from build123d import *

# Parameters (mm, degrees)
SKETCH1_R               = 18
BOSS_EXTRUDE1_DEPTH     = 7.5
CUT_EXTRUDE1_DEPTH      = 8.5
SKETCH3_R               = 6
BOSS_EXTRUDE2_DEPTH     = 2
SKETCH3_3_W             = 2.25
SKETCH3_3_H             = 1.5
CUT_EXTRUDE2_DEPTH      = 3
CUT_EXTRUDE2_DEPTH_BACK = 16
CIRPATTERN1_COUNT       = 16


with BuildPart() as part:
    # Sketch1 → Boss-Extrude1 (new body, symmetric)
    with BuildSketch(Plane.XY):
        Circle(SKETCH1_R)
    extrude(amount=BOSS_EXTRUDE1_DEPTH, both=True)

    # Sketch2 → Cut-Extrude1 (cut, symmetric)
    with BuildSketch(Plane.XY):
        with BuildLine():
            ThreePointArc((-2.51847991, 17.822941927), (-1.502149502, 15.735029188), (-1.035799814, 13.460205004))
            ThreePointArc((-1.035799814, 13.460205004), (0, 13.5), (1.035799814, 13.460205004))
            ThreePointArc((1.035799814, 13.460205004), (1.502149502, 15.735029188), (2.51847991, 17.822941927))
            ThreePointArc((2.51847991, 17.822941927), (0, 18), (-2.51847991, 17.822941927))
        make_face()
    cut_extrude1 = extrude(amount=CUT_EXTRUDE1_DEPTH, both=True, mode=Mode.SUBTRACT)

    # Sketch3 → Boss-Extrude2 (add)
    with BuildSketch(Plane.XY.offset(7.5)):
        Circle(SKETCH3_R)
        with BuildLine():
            ThreePointArc((1.125, 4.357106264), (0, -4.5), (-1.125, 4.357106264))
            Line((-1.125, 4.357106264), (-1.125, 5.107106264))
            Line((-1.125, 5.107106264), (1.125, 5.107106264))
            Line((1.125, 5.107106264), (1.125, 4.357106264))
        make_face(mode=Mode.SUBTRACT)
    extrude(amount=BOSS_EXTRUDE2_DEPTH)

    # Sketch3<3> → Cut-Extrude2 (cut, two sides)
    with BuildSketch(Plane.XY.offset(7.5)) as cut_extrude2_sk:
        with BuildLine():
            Line((1.125, 3.607106264), (-1.125, 3.607106264))
            Line((-1.125, 3.607106264), (-1.125, 4.357106264))
            ThreePointArc((-1.125, 4.357106264), (0, -4.5), (1.125, 4.357106264))
            Line((1.125, 4.357106264), (1.125, 3.607106264))
        make_face()
        with Locations((0, 4.357106264)):
            Rectangle(SKETCH3_3_W, SKETCH3_3_H)
    extrude(amount=CUT_EXTRUDE2_DEPTH, mode=Mode.SUBTRACT)
    extrude(cut_extrude2_sk.sketch, amount=-CUT_EXTRUDE2_DEPTH_BACK, mode=Mode.SUBTRACT)

    # CirPattern1: Cut-Extrude1 ×16 about axis
    cirpattern1_axis = Axis((0, 0, 0), (0, 0, 1))
    for i in range(1, CIRPATTERN1_COUNT):
        add(cut_extrude1.rotate(cirpattern1_axis, i * 360 / CIRPATTERN1_COUNT), mode=Mode.SUBTRACT)


solid = part.part
Build history of the part. All positions in model axes, mm. A direction names the side the tool comes from. Coordinates: 2 decimals unless noted, no trailing zeros. Write each loop counter-clockwise with the first axis right and the second up, starting at its lowest first coordinate (ties: lowest second). Pieces come first, ordered by that corner, then holes.
(1) Cut at B-B on y = 0. List the corners of the cut face in (x, z).
(2) Drill centre lines: line 1 (Y direction, x = 9, z = -6.5); line 2 (Y direction, x = -14, z = 2.75); line 3 (X direction, y = -13, z = 3.25). Where is each one in solid material? Low to high.
(3) Mould opens along Y. For faces 6 (the cylindrical face through (15.766, 1.513, 0.105)), 7 (the cylindrical face through (0, -13.5, 0.1)), 8 (the cylindrical face through (15.145, -4.636, 0.105)), 9 (the cylindrical face through (-9.989, 14.974, 0.105)) say: pulls with the +Y half, pulls with the -Y half, needs draft (parallel to the pull), parting line crosses it, or undercut.
(4) Cut at A-A on x = 0. List the corners of the cut face in (y, z), and give its area (3 significant figures).
(5) Cut at C-C on x = -15. List the corners of the cut face in (y, z), and give its area (3 significant figures).
(6) Pin check, flat tips, straight feed: pin 1 Ø1.5 at (x, z) = (8.5, 1.5) entering from -Y; pin 2 Ø3 at (y, z) = (13.5, 5.5) entering from -X; pin 3 Ø8 at (y, z) = (14, 2) entering from -X; pin 4 Ø1 at (x, y) = (-10.5, -10.5) entering from +Z. Stop position of each tip, or through.
(7) 3-axis set-ups, long thin cutter, end or side, ignore diameter. For faces 1 (the cylindrical face through (-6, 0, 8)), 2 (the cylindrical face through (-5.18, 12.467, 0.105)), 3 (the cylindrical face through (-13.987, -7.431, 0.105)), 4 (the flat face through (4, 4, -7.5)), 5 (the cylindrical face through (1.513, -15.766, 0.105)): which of +Z, -Z, +X, -X, +Y, -Y reach the whole face in a straight line?
Working result:
1. outline: (-13.5, -7.5) - (-4.5, -7.5) - (-4.5, 9.5) - (-6, 9.5) - (-6, 7.5) - (-13.5, 7.5) - close; (4.5, -7.5) - (13.5, -7.5) - (13.5, 7.5) - (6, 7.5) - (6, 9.5) - (4.5, 9.5) - close
2. line 1: y = -15.4 to -10.51, -10.06 to 10.06, 10.51 to 15.4
2. line 2: y = -10.73 to -7.44, -4.49 to -1.09, 1.09 to 4.49, 7.44 to 10.73
2. line 3: x = -10.42 to -6.67, -4.25 to 4.25, 6.67 to 10.42
3. face 6: undercut
3. face 7: pulls with the -Y half
3. face 8: undercut
3. face 9: pulls with the +Y half
4. outline: (-13.5, -7.5) - (-4.5, -7.5) - (-4.5, 9.5) - (-6, 9.5) - (-6, 7.5) - (-13.5, 7.5) - close; (5.11, -7.5) - (13.5, -7.5) - (13.5, 7.5) - (6, 7.5) - (6, 9.5) - (5.11, 9.5) - close
4. area: 266 mm2
5. outline: (-9.95, -7.5) - (-8.48, -7.5) - (-8.48, 7.5) - (-9.95, 7.5) - close; (-4.63, -7.5) - (-1.29, -7.5) - (-1.29, 7.5) - (-4.63, 7.5) - close; (1.29, -7.5) - (4.63, -7.5) - (4.63, 7.5) - (1.29, 7.5) - close; (8.48, -7.5) - (9.95, -7.5) - (9.95, 7.5) - (8.48, 7.5) - close
5. area: 144 mm2
6. pin 1: stops at y = -15.5
6. pin 2: stops at x = -10.82
6. pin 3: stops at x = -14.97
6. pin 4: passes through
7. face 1: +Z
7. face 2: +Z, -Z
7. face 3: +Z, -Z, -X
7. face 4: -Z, +X, -X, +Y, -Y
7. face 5: +Z, -Z, -Y
